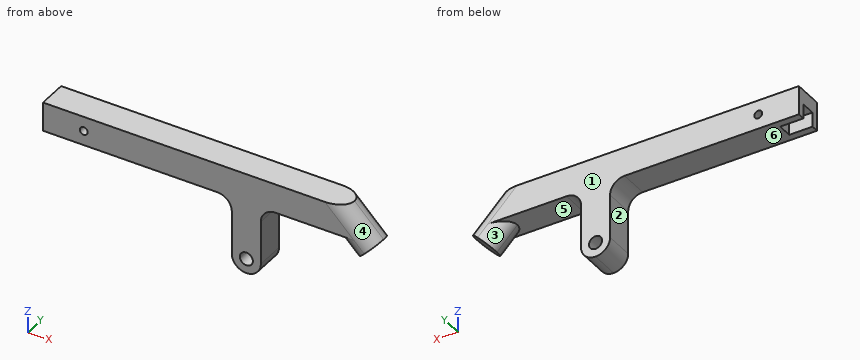
Solid Edge part; units mm, degrees
sketch "Sketch1" plane through (0, 0, 0) normal (0, -1, 0) x (1, 0, 0)
  line L0 (0, 25) -> (7.0711, 17.9289)
  line L1 (14.1421, 25) -> (7.0711, 17.9289)
  line L2 (4.1421, 35) -> (14.1421, 25)
  line L3 (4.1421, 35) -> (-100, 35)
  line L4 (-100, 35) -> (-100, 25)
  line L5 (-100, 25) -> (-35, 25)
  line L6 (-35, 25) -> (-35, 0)
  line L7 (-35, 0) -> (-25, 0)
  line L8 (-25, 0) -> (-25, 25)
  line L9 (-25, 25) -> (0, 25)
extrude "Protrusion1" add sketch "Sketch1" along normal mid plane 10
fillet "Round_1" radius 5 4 edges at (3.5355, -5, 21.4645) (3.5355, 5, 21.4645) (9.1421, 5, 30) (9.1421, -5, 30)
sketch "Sketch2" plane through (-61.4645, -5, 24) normal (0, -1, 0) x (1, 0, 0)
  circle A0 centre (31.4645, -19) radius 2.25
extrude "ExtrudedCutout_1" cut sketch "Sketch2" along normal mid plane 69.4908
fillet "Round_2" radius 5 4 edges at (-25, 0, 0) (-35, 0, 0) (-25, 0, 25) (-35, 0, 25)
sketch "Sketch3" plane through (-100, 0, 43) normal (-1, 0, 0) x (0, 0, -1)
  line L0 (18, -2.5) -> (13, -2.5)
  line L1 (13, -2.5) -> (13, 2.5)
  line L2 (13, 2.5) -> (18, 2.5)
  line L3 (18, 2.5) -> (18, -2.5)
extrude "ExtrudedCutout_2" cut sketch "Sketch3" against normal blind 8
sketch "Sketch4" plane through (0, 0, 0) normal (0, -1, 0) x (1, 0, 0)
  circle A0 centre (-86, 30) radius 1.35
extrude "ExtrudedCutout_3" cut sketch "Sketch4" along normal mid plane 29.2691
properties material "PVC"
Model file for the job. Use its own axes, mm. Face numbers are marked on the shaded views. A direction names the side the tool comes from. Give positions to 0.01 mm unless a question says otherwise; leave off trailing zeros. Loops run counter-clockwise (first coordinate to the right, second up) from the corner with the lowest first, then second, coordinate; pieces in that order, holes last. Notation, with made-up numbers: (29, 47) -> (73, 47) arc R17 ccw to (73, 51) -> close; hole circle Ø8 at (14.25, 19). An arc over 180 degrees is marked (long way). Use a Markdown table: item, result. Add a question column.
(1) Wall check: line 1 along Z through (x, y) = (-86, 1.25); line 2 along Z through (x, y) = (-84, 4); line 3 along Z through (x, y) = (-30, -0.25). Give the ranges that are in metal, low to high.
(2) Mould opens along X. For the marked faces 4, 5 and 6 say: +X half, -X half, draft (parallel to the pull), parting line (faces both ways), or undercut.
(3) Tool access for the marked faces 1, 2 and 3: list every direction of +Z, -Z, +X, -X, +Y, -Y with a clear straight run to the whole face (end or side of a thin tool).
(4) Slice it at C-C on z = 15. List the corners of the cut face in (x, y), and give its area (3 significant figures).
(5) Drop flat-ended pins along their axis: pin 1 Ø3 at (y, z) = (0, 24) entering from -X; pin 2 Ø5 at (y, z) = (-1, 9.5) entering from +X; pin 3 Ø2.5 at (x, z) = (-86, 30) entering from +Y; pin 4 Ø1 at (y, z) = (-1, 26.5) entering from +X. Give the stop position or say it passes through.
(6) Slice it at D-D on x = -12. List the corners of the cut face in (y, z).
(7) Slice it at B-B on y = -4. Give the number of separate pieces and of enclosed holes in the cut face, and give its area (3 significant figures).
(8) Slice it at A-A on x = -86. List the corners of the cut face in (y, z), and give its area (3 significant figures).
Filled sheet:
| question | item | result |
|---|---|---|
| 1 | line 1 | 25 to 28.65, 31.35 to 35 |
| 1 | line 2 | 25 to 35 |
| 1 | line 3 | 0 to 2.75, 7.25 to 35 |
| 2 | face 4 | +X half |
| 2 | face 5 | undercut |
| 2 | face 6 | draft |
| 3 | face 1 | +Z, -Z, +X, -X, +Y |
| 3 | face 2 | -Z, -X, +Y, -Y |
| 3 | face 3 | -Z, +Y |
| 4 | outline | (-35, -5) -> (-25, -5) -> (-25, 5) -> (-35, 5) -> close |
| 4 | area | 100 mm2 |
| 5 | pin 1 | x = -92 |
| 5 | pin 2 | x = -25 |
| 5 | pin 3 | through |
| 5 | pin 4 | x = 13.02 |
| 6 | outline | (-5, 25) -> (5, 25) -> (5, 35) -> (-5, 35) -> close |
| 7 | separate pieces | 1 |
| 7 | enclosed holes | 2 |
| 7 | area | 1,320 mm2 |
| 8 | outline | (-5, 25) -> (5, 25) -> (5, 28.65) -> (-5, 28.65) -> close; (-5, 31.35) -> (5, 31.35) -> (5, 35) -> (-5, 35) -> close |
| 8 | area | 73.0 mm2 |
